```python
from build123d import *

# Parameters (mm, degrees)
SKETCH1_R               = 15.875
SKETCH1_R_2             = 3.175
BOSS_EXTRUDE1_DEPTH     = 2.116666667
SKETCH2_R               = 1.5875
CUT_EXTRUDE1_DEPTH      = 3.116666667
CUT_EXTRUDE1_DEPTH_BACK = 3.116666667


with BuildPart() as part:
    # Sketch1 → Boss-Extrude1 (new body, symmetric)
    with BuildSketch(Plane(origin=(0, 0, 0), x_dir=(1, 0, 0), z_dir=(0, 1, 0))):
        Circle(SKETCH1_R)
        Circle(SKETCH1_R_2, mode=Mode.SUBTRACT)
    extrude(amount=BOSS_EXTRUDE1_DEPTH, both=True)

    # Sketch2 → Cut-Extrude1 (cut, two sides)
    with BuildSketch(Plane(origin=(0, 0, 0), x_dir=(1, 0, 0), z_dir=(0, 1, 0))) as cut_extrude1_sk:
        with Locations((0, 9.525)):
            Circle(SKETCH2_R)
        with Locations((8.248891971, 4.7625)):
            Circle(SKETCH2_R)
        with Locations((8.248891971, -4.7625)):
            Circle(SKETCH2_R)
        with Locations((0, -9.525)):
            Circle(SKETCH2_R)
        with Locations((-8.248891971, -4.7625)):
            Circle(SKETCH2_R)
        with Locations((-8.248891971, 4.7625)):
            Circle(SKETCH2_R)
    extrude(amount=CUT_EXTRUDE1_DEPTH, mode=Mode.SUBTRACT)
    extrude(cut_extrude1_sk.sketch, amount=-CUT_EXTRUDE1_DEPTH_BACK, mode=Mode.SUBTRACT)


solid = part.part
```
Source: CAD feature listing. Evaluate the final solid. Frame: model axes, mm. Give positions to 0.01 mm unless a question says otherwise; leave off trailing zeros. Write each loop counter-clockwise with the first axis right and the second up, starting at its lowest first coordinate (ties: lowest second). Pieces come first, ordered by that corner, then holes.
1. Section query D-D (z = -10). Return the cut outline in (x, y).
2. Section query A-A (z = 0). Return the cut outline in (x, y) (3 decimals).
3. Material intervals for line 1 along Z through (x, y) = (0, 1) (1 decimal); line 2 along Z through (x, y) = (-1, 1.65); line 3 along Z through (x, y) = (-8, -1.75), sorted ascending.
4. Section query B-B (x = 0). Return the cut outline in (y, z) (1 decimal).
5. Section query C-C (y = -0.7). Count the separate pieces of the cut face and the enclosed holes in it, then the cut area to 3 significant figures.
6. First-contact query: pin 1 (1 mm diameter, centred on x = -1, y = -1.5, fed in from +Z); pin 2 (1.5 mm diameter, centred on y = -0.5, z = 4, fed in from +X); pin 3 (1.9 mm diameter, centred on x = -8.25, z = -4.76, fed in from -Y); pin 4 (1 mm diameter, centred on y = -0.5, z = 7.5, fed in from +X). Flat tips, straight axial feed; report the tip coordinate or a pass-through.
7. Pull-direction query (Z, two-part tool) for faces 1 (the face through (0, 2.117, -4)), 2 (the face through (-9.835, 0.03, 4.693)), 3 (the face through (-3.441, 0.03, 15.497)); classes: +Z half, -Z half, draft (parallel to the pull), parting line (faces both ways), or undercut.
Output values:
1. outline: (-12.33, -2.12) - (-1.51, -2.12) - (-1.51, 2.12) - (-12.33, 2.12) - close; (1.51, -2.12) - (12.33, -2.12) - (12.33, 2.12) - (1.51, 2.12) - close
2. outline: (-15.875, -2.117) - (-3.175, -2.117) - (-3.175, 2.117) - (-15.875, 2.117) - close; (3.175, -2.117) - (15.875, -2.117) - (15.875, 2.117) - (3.175, 2.117) - close
3. line 1: z = -15.9 to -11.1, -7.9 to -3.2, 3.2 to 7.9, 11.1 to 15.9
3. line 2: z = -15.84 to -10.76, -8.29 to -3.01, 3.01 to 8.29, 10.76 to 15.84
3. line 3: z = -13.71 to -6.33, -3.19 to 3.19, 6.33 to 13.71
4. outline: (-2.1, -15.9) - (2.1, -15.9) - (2.1, -11.1) - (-2.1, -11.1) - close; (-2.1, -7.9) - (2.1, -7.9) - (2.1, -3.2) - (-2.1, -3.2) - close; (-2.1, 3.2) - (2.1, 3.2) - (2.1, 7.9) - (-2.1, 7.9) - close; (-2.1, 11.1) - (2.1, 11.1) - (2.1, 15.9) - (-2.1, 15.9) - close
5. separate pieces: 1
5. enclosed holes: 7
5. area: 713 mm2
6. pin 1: stops at z = 15.87
6. pin 2: stops at x = 15.54
6. pin 3: passes through
6. pin 4: stops at x = 14.25
7. face 1: draft
7. face 2: undercut
7. face 3: parting line
